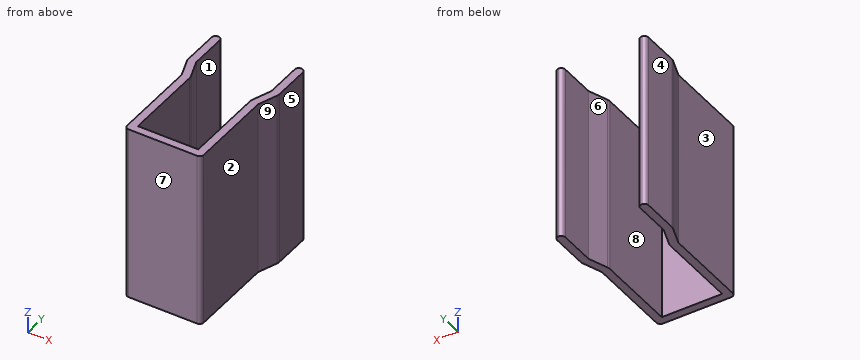
```python
from build123d import *

# Parameters (mm, degrees)
F0_W     = 1.6
F0_H     = 8
F1_DEPTH = 35
F2_R     = 0.79999


# Not quite as in the source:
# - a fillet or chamfer is up to 0.001 mm smaller than in the source, because OpenCascade refuses the exact size


with BuildPart() as f1:
    # F0 (on Top) → F1 (new body)
    with BuildSketch(Plane.XY):
        Polygon((0, 16), (0, 0), (-12, 0), (-12, 16), (-13.6, 16), (-13.6, -1.6), (1.6, -1.6), (1.6, 16), align=None)
        with BuildLine():
            ThreePointArc((0.0964918067, 16.5472322293), (0.0243075952, 16.2778370843), (0, 16))
            Line((0, 16), (1.6, 16))
            Line((1.6, 16), (0.0964918067, 16.5472322293))
        make_face()
        with BuildLine():
            Line((-13.6, 16), (-12, 16))
            ThreePointArc((-12, 16), (-12.0243075952, 16.2778370843), (-12.0964918067, 16.5472322293))
            Line((-12.0964918067, 16.5472322293), (-13.6, 16))
        make_face()
        Polygon((0.0964918067, 16.5472322293), (1.6, 16), (2.9680805733, 19.7587704831), (1.46457238, 20.3060027125), align=None)
        Polygon((-14.9680805733, 19.7587704831), (-13.6, 16), (-12.0964918067, 16.5472322293), (-13.46457238, 20.3060027125), align=None)
        with BuildLine():
            Line((1.46457238, 20.3060027125), (2.9680805733, 19.7587704831))
            ThreePointArc((2.9680805733, 19.7587704831), (3.0402647849, 20.0281656282), (3.06457238, 20.3060027125))
            Line((3.06457238, 20.3060027125), (1.46457238, 20.3060027125))
        make_face()
        with Locations((2.26457238, 24.3060027125)):
            Rectangle(F0_W, F0_H)
        with BuildLine():
            ThreePointArc((-15.06457238, 20.3060027125), (-15.0402647849, 20.0281656282), (-14.9680805733, 19.7587704831))
            Line((-14.9680805733, 19.7587704831), (-13.46457238, 20.3060027125))
            Line((-13.46457238, 20.3060027125), (-15.06457238, 20.3060027125))
        make_face()
        with Locations((-14.26457238, 24.3060027125)):
            Rectangle(F0_W, F0_H)
    extrude(amount=F1_DEPTH)

    # F2 (radius 0.8 in the source; OpenCascade refuses exactly that, so slightly less here)
    f2_edges = [f1.edges().sort_by_distance(p)[0] for p in [
        (1.6, -1.6, 17.5),
        (-13.6, -1.6, 17.5),
        (-15.064572, 28.306003, 17.5),
        (3.064572, 28.306003, 17.5),
        (1.464572, 28.306003, 17.5),
        (-13.464572, 28.306003, 17.5),
    ]]
    fillet(f2_edges, radius=F2_R)


solid = f1.part
```
The model under review builds one solid part; all positions refer to its coordinate system, in mm. Face numbers are marked on the shaded views. A direction names the side the tool comes from. Round coordinates to 2 decimals unless told otherwise and drop trailing zeros. Loops run counter-clockwise (first coordinate to the right, second up) from the corner with the lowest first, then second, coordinate; pieces in that order, holes last. Notation, with made-up numbers: (38, 49) -> (46, 49) arc R28 ccw to (46, 85) -> close; hole circle Ø3 at (77.25, 21.25). An arc over 180 degrees is marked (long way). Answer as a JSON object with one key per item and string values. Group by question number.
1) For line 1 (X direction, y = 11, z = 6); line 2 (X direction, y = 22.25, z = 18); line 3 (Y direction, x = -10.25, z = 17), list the stretches that pass through material, from the lowest coordinate up. Write a range as [from, to].
2) Mouldability with a two-part tool opening along X and no side actions: class the marked faces 6, 7, 8 and 9 as released by +X, released by -X, zero draft, split by the parting line, or undercut.
3) For the marked faces 1, 2, 3, 4 and 5, list the 3-axis set-ups (+Z, -Z, +X, -X, +Y, -Y) from which the entire face can be reached by the end or side of a thin tool; tool diameter is ignored.
4) For pin 1 Ø13 at (y, z) = (7, 23.5) entering from -X; pin 2 Ø5 at (y, z) = (9.5, 21.5) entering from +X; pin 3 Ø8 at (x, z) = (-7, 8.5) entering from +Y, all flat-tipped, find the tip position at first contact; note any pin that passes through.
5) We need section D-D on y = 18. Write out the cut boundary in (x, z), then the cut area to 3 significant figures.
6) We need section A-A on y = 2.75. Write out the cut boundary in (x, z).
7) We need section C-C on x = -3.25. Write out the cut boundary in (y, z).
Result set:
{
 "1": {"line 1": "[-13.6, -12], [0, 1.6]", "line 2": "[-15.06, -13.46], [1.46, 3.06]", "line 3": "[-1.6, 0]"},
 "2": {"face 6": "undercut", "face 7": "zero draft", "face 8": "undercut", "face 9": "released by +X"},
 "3": {"face 1": "+Z, -Z, +Y", "face 2": "+Z, -Z, +X, -Y", "face 3": "+Z, -Z, -X, -Y", "face 4": "+Z, -Z, -X, +Y, -Y", "face 5": "+Z, -Z, +X, +Y, -Y"},
 "4": {"pin 1": "x = -13.6", "pin 2": "x = 1.6", "pin 3": "y = 0"},
 "5": {"outline": "(-14.33, 0) -> (-12.63, 0) -> (-12.63, 35) -> (-14.33, 35) -> close; (0.63, 0) -> (2.33, 0) -> (2.33, 35) -> (0.63, 35) -> close", "area": "119 mm²"},
 "6": {"outline": "(-13.6, 0) -> (-12, 0) -> (-12, 35) -> (-13.6, 35) -> close; (0, 0) -> (1.6, 0) -> (1.6, 35) -> (0, 35) -> close"},
 "7": {"outline": "(-1.6, 0) -> (0, 0) -> (0, 35) -> (-1.6, 35) -> close"}
}
